```python
from build123d import *

# Parameters (mm, degrees)
CROQUIS1_R              = 1
SALIENTE_EXTRUIR1_DEPTH = 6
CROQUIS2_W              = 9
CROQUIS2_H              = 2
CORTAR_EXTRUIR1_DEPTH   = 8
REDONDEO1_R             = 4.5
REDONDEO2_R             = 3
CORTAR_EXTRUIR2_DEPTH   = 43.66438796


# Some blends are built 0.0001 mm under size
with BuildPart() as part:
    # Croquis1 → Saliente-Extruir1 (new body)
    with BuildSketch(Plane.XY):
        with BuildLine():
            Line((-4.5, -1.5), (-1.609347694, -1.5))
            ThreePointArc((-1.609347694, -1.5), (0, 2.2), (1.609347694, -1.5))
            Line((1.609347694, -1.5), (4.5, -1.5))
            Line((4.5, -1.5), (4.5, 42))
            Line((4.5, 42), (-4.5, 42))
            Line((-4.5, 42), (-4.5, -1.5))
        make_face()
        with Locations((0, 38.5)):
            Circle(CROQUIS1_R, mode=Mode.SUBTRACT)
    extrude(amount=SALIENTE_EXTRUIR1_DEPTH)

    # Croquis2 → Cortar-Extruir1 (cut)
    with BuildSketch(Plane(origin=(0, 42, 0), x_dir=(1, 0, 0), z_dir=(0, 1, 0))):
        with Locations((0, -3)):
            Rectangle(CROQUIS2_W, CROQUIS2_H)
    extrude(amount=-CORTAR_EXTRUIR1_DEPTH, mode=Mode.SUBTRACT)

    # Redondeo1
    redondeo1_edges = [part.edges().sort_by_distance(p)[0] for p in [
        (-4.5, 34, 3),
        (4.5, 34, 3),
    ]]
    fillet(redondeo1_edges, radius=REDONDEO1_R - 0.0001)  # a hair under: the kernel refuses the full size

    # Redondeo2
    # the kernel refuses this fillet: 3 mm, written as the material it takes off along each edge
    with BuildSketch(Plane(origin=(-4.5, 42, -3.5), x_dir=(0, -1, 0), z_dir=(0, 0, 1)), Plane(origin=(-4.5, 42, -7.5), x_dir=(0, -1, 0), z_dir=(0, 0, 1))) as redondeo2_piece_1:
        with BuildLine():
            CenterArc((REDONDEO2_R, REDONDEO2_R), REDONDEO2_R, 180, 90)
            Line((0, REDONDEO2_R), (-REDONDEO2_R * 0.02, REDONDEO2_R))
            Line((-REDONDEO2_R * 0.02, REDONDEO2_R), (-REDONDEO2_R * 0.02, -REDONDEO2_R * 0.02))
            Line((-REDONDEO2_R * 0.02, -REDONDEO2_R * 0.02), (REDONDEO2_R, -REDONDEO2_R * 0.02))
            Line((REDONDEO2_R, -REDONDEO2_R * 0.02), (REDONDEO2_R, 0))
        make_face()
    extrude(amount=17, mode=Mode.SUBTRACT)
    with BuildSketch(Plane(origin=(4.5, 42, -7.5), x_dir=(0, -1, 0), z_dir=(0, 0, 1)), Plane(origin=(4.5, 42, -3.5), x_dir=(0, -1, 0), z_dir=(0, 0, 1))) as redondeo2_piece_2:
        with BuildLine():
            CenterArc((REDONDEO2_R, -REDONDEO2_R), REDONDEO2_R, 90, 90)
            Line((0, -REDONDEO2_R), (-REDONDEO2_R * 0.02, -REDONDEO2_R))
            Line((-REDONDEO2_R * 0.02, -REDONDEO2_R), (-REDONDEO2_R * 0.02, REDONDEO2_R * 0.02))
            Line((-REDONDEO2_R * 0.02, REDONDEO2_R * 0.02), (REDONDEO2_R, REDONDEO2_R * 0.02))
            Line((REDONDEO2_R, REDONDEO2_R * 0.02), (REDONDEO2_R, 0))
        make_face()
    extrude(amount=17, mode=Mode.SUBTRACT)
    with BuildSketch(Plane(origin=(4.5, -1.5, -7.495016295), x_dir=(0, 1, 0), z_dir=(0, 0, 1))) as redondeo2_piece_3:
        with BuildLine():
            CenterArc((2.998006518, 3), REDONDEO2_R, 182.088849817, 87.911150183)
            Line((0, 2.890652306), (-0.05996013, 2.888465352))
            ThreePointArc((-0.05996013, 2.888465352), (-0.06, 1.445326153), (-0.06, 0))
            Line((-0.06, 0), (0, -0.06))
            Line((0, -0.06), (2.998006518, -0.06))
            Line((2.998006518, -0.06), (2.998006518, 0))
        make_face()
    extrude(amount=20.99003259, mode=Mode.SUBTRACT)
    with BuildSketch(Plane(origin=(-4.5, -1.5, -7.495016295), x_dir=(0, 1, 0), z_dir=(0, 0, 1))) as redondeo2_piece_4:
        with BuildLine():
            CenterArc((2.998006518, -3), REDONDEO2_R, 90, 87.911150183)
            Line((0, -2.890652306), (-0.05996013, -2.888465352))
            ThreePointArc((-0.05996013, -2.888465352), (-0.06, -1.445326153), (-0.06, 0))
            Line((-0.06, 0), (0, 0.06))
            Line((0, 0.06), (2.998006518, 0.06))
            Line((2.998006518, 0.06), (2.998006518, 0))
        make_face()
    extrude(amount=20.99003259, mode=Mode.SUBTRACT)

    # Croquis3 → Cortar-Extruir2 (cut, through all)
    with BuildSketch(Plane.XY.offset(6)):
        with BuildLine():
            Line((-3, 8), (-3, 29.5))
            ThreePointArc((-3, 29.5), (0, 32.5), (3, 29.5))
            Line((3, 29.5), (3, 8))
            ThreePointArc((3, 8), (0, 5), (-3, 8))
        make_face()
    extrude(amount=-CORTAR_EXTRUIR2_DEPTH, mode=Mode.SUBTRACT)


solid = part.part
```
Can you work these out from the model? Positions are in its coordinate system, mm. A direction names the side the tool comes from. Round coordinates to 2 decimals unless told otherwise and drop trailing zeros. Loops run counter-clockwise (first coordinate to the right, second up) from the corner with the lowest first, then second, coordinate; pieces in that order, holes last.
Item 1: Please list where these lines run through material, in increasing order: L1, parallel to X at y = 27, z = 3.45; L2, parallel to Y at x = 0, z = 5.1; L3, parallel to Z at x = -3, y = 37.5.
Item 2: Which directions (+Z, -Z, +X, -X, +Y, -Y) give clear straight access to the entire face, cutting with the end or side of a thin tool? Please do faces 4 (the flat face through (3, 19, 3)), 5 (the cylindrical face through (-3.682, -0.561, 2.958)), 6 (the cylindrical face through (3.147, 32.717, 2.986)).
Item 3: Suppose I cut it at A-A, the plane y = 24. Write out the boundary of the cut face in (x, z), then the cut area to 3 significant figures.
Item 4: Suppose I cut it at D-D, the plane y = 38.5. Write out the boundary of the cut face in (x, z).
Item 5: If we mould it in two halves opening along Y, with no side actions, what happens to faces 1 (the cylindrical face through (-3.6, 41.14, 4.99)), 2 (the cylindrical face through (-0.1, 32.5, 3)), 3 (the flat face through (-4, 25, 0))? For each: +Y half, -Y half, draft (parallel to the pull), parting line (faces both ways), or undercut.
Item 6: Will these pins go through, and if not, where does the flat tip stop? pin 1 Ø1.8 at (x, y) = (0, 38.5) entering from +Z; pin 2 Ø1.5 at (y, z) = (32.5, 3) entering from -X.
Item 7: Suppose I cut it at B-B, the plane z = 4.45. Write out the boundary of the cut face in (x, y), then the cut area to 3 significant figures.
Reported:
1. L1: x = -4.5 to -3, 3 to 4.5
1. L2: y = 2.2 to 5, 32.5 to 37.5, 39.5 to 42
1. L3: z = 0 to 2, 4 to 6
2. face 4: +Z, -Z
2. face 5: +Z, -Z, -X, -Y
2. face 6: +X, +Y
3. outline: (-4.5, 0) - (-3, 0) - (-3, 6) - (-4.5, 6) - close; (3, 0) - (4.5, 0) - (4.5, 6) - (3, 6) - close
3. area: 18.0 mm2
4. outline: (-4.5, 0) - (-1, 0) - (-1, 2) - (-4.5, 2) - close; (-4.5, 4) - (-1, 4) - (-1, 6) - (-4.5, 6) - close; (1, 0) - (4.5, 0) - (4.5, 2) - (1, 2) - close; (1, 4) - (4.5, 4) - (4.5, 6) - (1, 6) - close
5. face 1: +Y half
5. face 2: undercut
5. face 3: draft
6. pin 1: passes through
6. pin 2: stops at x = -3.9
7. outline: (-4.5, 1.5) arc R3 ccw to (-1.61, -1.5) arc R2.2 cw (long way) to (1.61, -1.5) arc R3 ccw to (4.5, 1.5) - (4.5, 39) arc R3 ccw to (1.5, 42) - (-1.5, 42) arc R3 ccw to (-4.5, 39) - close; hole (-3, 8) arc R3 ccw to (3, 8) - (3, 29.5) arc R3 ccw to (-3, 29.5) - close; hole circle Ø2 at (0, 38.5)
7. area: 210 mm2
